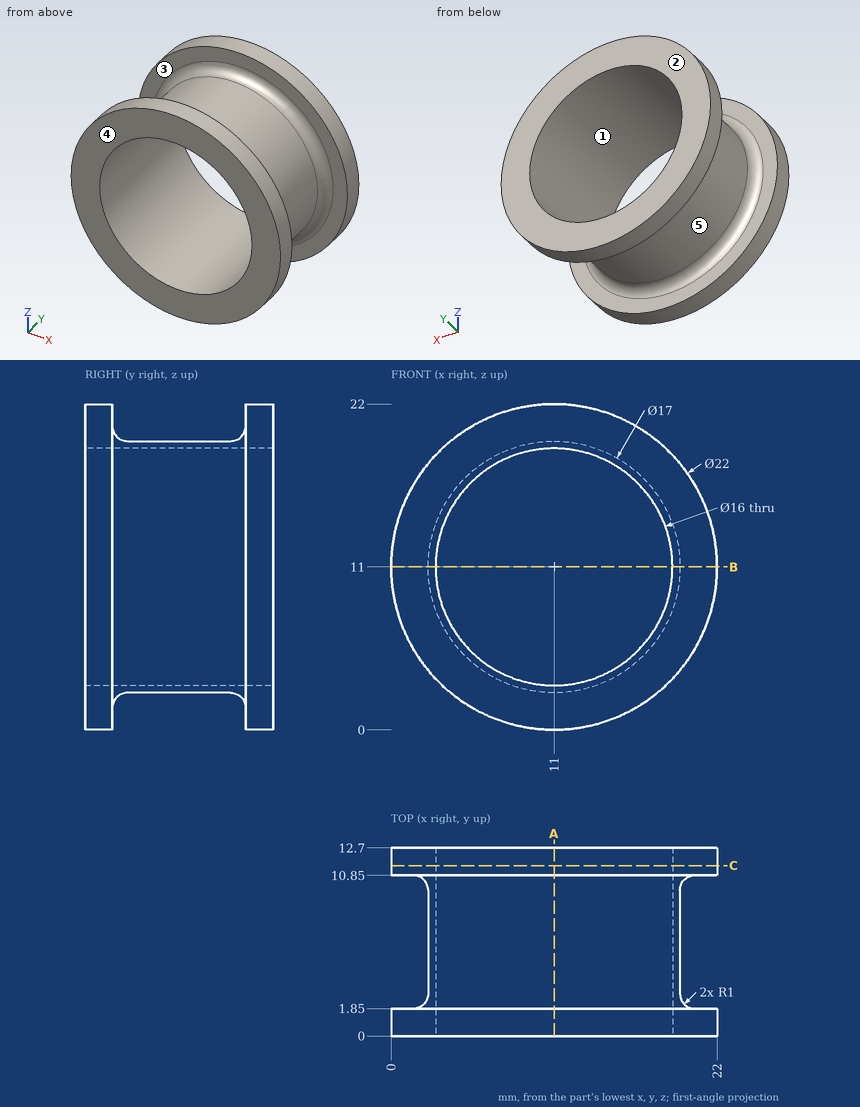
Check sheet for the drawn part. Datum: minimum x, y, z corner. Units: mm. A direction names the side the tool comes from. Give positions to 0.01 mm unless a question says otherwise; leave off trailing zeros. Order: outer loops, then holes, each group sorted by start corner. A loop starts at its lowest first (then second) coordinate and runs counter-clockwise, first axis right, second up.
1. Access from +Z, -Z, +X, -X, +Y, -Y to the whole of each face (thin tool, end or side, straight path). Record for the marked faces 4 and 5.
Completed:
face 4: +Z, -Z, +X, -X, -Y
face 5: none
2. Sectioned sample at A-A (x = 11). Record the boundary of the cut face in (y, z).
Completed:
outline: (0, 0) - (1.85, 0) - (1.85, 1.5) arc R1 cw to (2.85, 2.5) - (9.85, 2.5) arc R1 cw to (10.85, 1.5) - (10.85, 0) - (12.7, 0) - (12.7, 3) - (0, 3) - close; (0, 19) - (12.7, 19) - (12.7, 22) - (10.85, 22) - (10.85, 20.5) arc R1 cw to (9.85, 19.5) - (2.85, 19.5) arc R1 cw to (1.85, 20.5) - (1.85, 22) - (0, 22) - close
3. Scan lines: line 1 (X direction, y = 4.5, z = 11); line 2 (Y direction, x = 1.75, z = 9). Record each from-to range of solid material in increasing order.
Completed:
line 1: x = 2.5 to 3, 19 to 19.5
line 2: y = 0 to 1.85, 10.85 to 12.7
4. Draft check along Y on the marked faces 1, 2 and 3. Enter one of: pulls with the +Y half, pulls with the -Y half, needs draft (parallel to the pull), parting line crosses it, or undercut.
Completed:
face 1: needs draft
face 2: pulls with the +Y half
face 3: undercut
5. Sectioned sample at B-B (z = 11). Record the boundary of the cut face in (x, y), then the cut area to 3 significant figures.
Completed:
outline: (0, 0) - (3, 0) - (3, 12.7) - (0, 12.7) - (0, 10.85) - (1.5, 10.85) arc R1 cw to (2.5, 9.85) - (2.5, 2.85) arc R1 cw to (1.5, 1.85) - (0, 1.85) - close; (19, 0) - (22, 0) - (22, 1.85) - (20.5, 1.85) arc R1 cw to (19.5, 2.85) - (19.5, 9.85) arc R1 cw to (20.5, 10.85) - (22, 10.85) - (22, 12.7) - (19, 12.7) - close
area: 32.1 mm2
6. Depth check by flat-ended pin: pin 1 (5 mm diameter, centred on x = 15.5, z = 11.5, fed in from +Y); pin 2 (2 mm diameter, centred on x = 11.5, y = 3.5, fed in from +Z); pin 3 (5 mm diameter, centred on x = 5, y = 2.5, fed in from +Z); pin 4 (4 mm diameter, centred on x = 5.5, y = 9, fed in from +Z). Enter the tip coordinate at first touch or a pass-through.
Completed:
pin 1: passes through
pin 2: stops at z = 19.55
pin 3: stops at z = 21.4
pin 4: stops at z = 20.93
7. Sectioned sample at C-C (y = 11.5). Record the boundary of the cut face in (x, z).
Completed:
outline: circle Ø22 at (11, 11); hole circle Ø16 at (11, 11)
